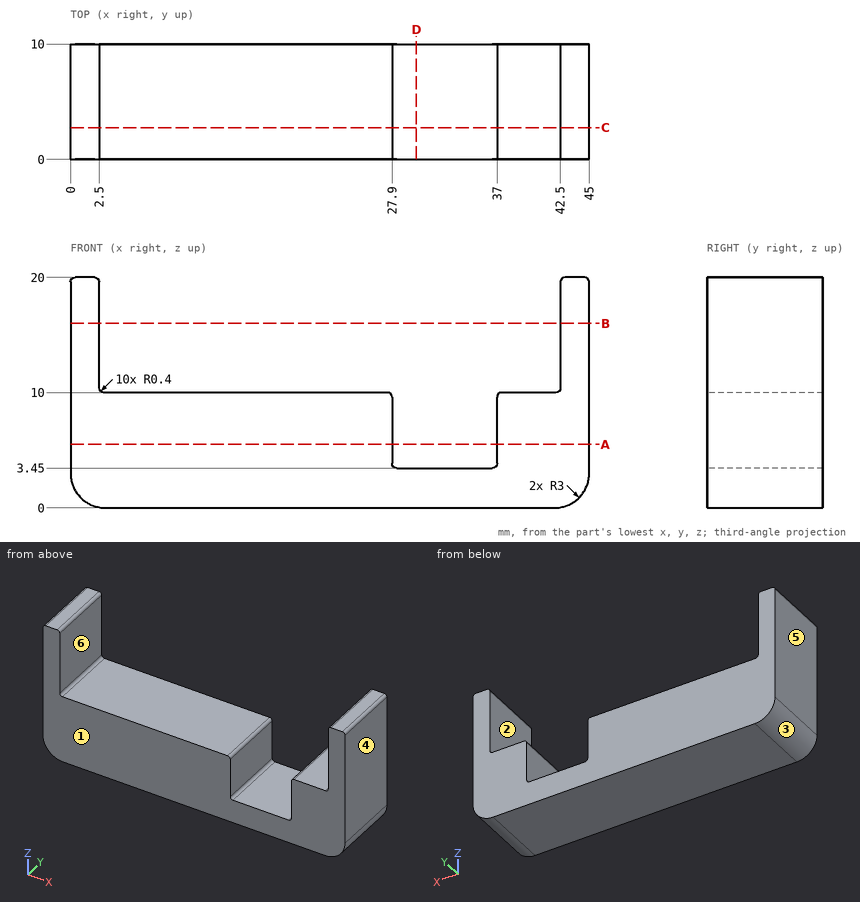
Input: dimensioned drawing with shaded views. Units: mm. Origin: part minimum x, y, z. A direction names the side the tool comes from. Give positions to 0.01 mm unless a question says otherwise; leave off trailing zeros. Write each loop counter-clockwise with the first axis right and the second up, starting at its lowest first coordinate (ties: lowest second). Pieces come first, ordered by that corner, then holes. Notation, with made-up numbers: (-16.75, 69) - (22.25, 69) arc R25 cw to (22.25, 101) - close; hole circle Ø2 at (-0.5, 87.5). An arc over 180 degrees is marked (long way). One line per item, written item: value. Start each with the question number.
Q1. Section query A-A, the plane z = 5.5. Return the cut outline in (x, y), then the cut area to 3 significant figures.
Q2. Section query C-C, the plane y = 2.75. Return the cut outline in (x, z), then the cut area to 3 significant figures.
Q3. Material intervals for probe 1 along X at (y, z) = (5, 11.25); probe 2 along X at (y, z) = (7.75, 7.5); probe 3 along Z at (x, y) = (42, 9), sorted ascending. Write a range as from..to.
Q4. First-contact query: pin 1 Ø1 at (x, y) = (12.5, 4.5) entering from -Z; pin 2 Ø5 at (x, y) = (11, 4) entering from +Z. Flat tips, straight axial feed; report the tip coordinate or a pass-through.
Q5. Set-up query: the marked faces 5 and 6. Return all of +Z, -Z, +X, -X, +Y, -Y with unobstructed straight access to the full face (end or side cutting, diameter ignored); none if empty.
Q6. Draft query along X for the marked faces 1, 2, 3 and 4. Return one class per face: +X half, -X half, draft (parallel to the pull), parting line (faces both ways), or undercut.
Q7. Section query D-D, the plane x = 30. Return the cut outline in (y, z), then the cut area to 3 significant figures.
Q8. Section query B-B, the plane z = 16. Return the cut outline in (x, y).
Answer:
1. outline: (0, 0) - (27.9, 0) - (27.9, 10) - (0, 10) - close; (37, 0) - (45, 0) - (45, 10) - (37, 10) - close
1. area: 359 mm2
2. outline: (0, 3) arc R3 ccw to (3, 0) - (42, 0) arc R3 ccw to (45, 3) - (45, 19.6) arc R0.4 ccw to (44.6, 20) - (42.9, 20) arc R0.4 ccw to (42.5, 19.6) - (42.5, 10.4) arc R0.4 cw to (42.1, 10) - (37.4, 10) arc R0.4 ccw to (37, 9.6) - (37, 3.85) arc R0.4 cw to (36.6, 3.45) - (28.3, 3.45) arc R0.4 cw to (27.9, 3.85) - (27.9, 9.6) arc R0.4 ccw to (27.5, 10) - (2.9, 10) arc R0.4 cw to (2.5, 10.4) - (2.5, 19.6) arc R0.4 ccw to (2.1, 20) - (0.4, 20) arc R0.4 ccw to (0, 19.6) - close
2. area: 436 mm2
3. probe 1: x = 0..2.5, 42.5..45
3. probe 2: x = 0..27.9, 37..45
3. probe 3: z = 0..10
4. pin 1: stops at z = 0
4. pin 2: stops at z = 10
5. face 5: +Z, -Z, -X, +Y, -Y
5. face 6: +Z, +Y, -Y
6. face 1: draft
6. face 2: undercut
6. face 3: -X half
6. face 4: +X half
7. outline: (0, 0) - (10, 0) - (10, 3.45) - (0, 3.45) - close
7. area: 34.5 mm2
8. outline: (0, 0) - (2.5, 0) - (2.5, 10) - (0, 10) - close; (42.5, 0) - (45, 0) - (45, 10) - (42.5, 10) - close
